The model under review builds one solid part; all positions refer to its coordinate system, in mm. A direction names the side the tool comes from. Coordinates: 2 decimals unless noted, no trailing zeros. Use one line per item in the form item = value. Start each with the question number.
(1) Insertion check: pin 1 Ø6 at (x, z) = (1, -8) entering from +Y; pin 2 Ø2 at (y, z) = (10, -5.5) entering from +X; pin 3 Ø1 at (x, y) = (-17, 7.5) entering from -Z (3 decimals); pin 4 Ø4 at (x, y) = (12.5, 8.5) entering from -Z. Each pin has a flat end and moves straight along its axis. Give the tip position at first contact, or say it passes through.
(2) For faces 5 (the cylindrical face through (-0.764, 0.724, 16.364)), 6 (the flat face through (-15.3, 10.795, 2.4)), 7 (the flat face through (0, 8, 16)), list the 3-axis set-ups (+Z, -Z, +X, -X, +Y, -Y) from which the entire face can be reached by the end or side of a thin tool; tool diameter is ignored.
(3) Take a section at A-A (x = -3.5). State how many separate pieces and enclosed holes the cut face has, then the cut area to 3 significant figures.
(4) Wall thickness on line 1 along X through (y, z) = (7.25, 6); line 2 along X through (y, z) = (7.5, 1.5); line 3 along Z through (x, y) = (-36, 6): over which ranges is each line inside the solid? List them lowest first.
(5) Mouldability with a two-part tool opening along Z and no side actions: class faces 1 (the flat face through (-39.597, 6.261, -10.359)), 2 (the cylindrical face through (-23.17, 0.72, 6.88)), 3 (the flat face through (-15.426, 6.261, -17.565)), 4 (the cylindrical face through (-15.374, 1.279, 3.601)) as +Z half, -Z half, draft (parallel to the pull), parting line (faces both ways), or undercut.
```python
from build123d import *

# Parameters (mm, degrees)
SKETCH1_W           = 16.825477707
SKETCH1_H           = 12.7
BOSS_EXTRUDE1_DEPTH = 12.7
FILLET1_R           = 7.62
SKETCH2_R           = 1.905
CUT_EXTRUDE1_DEPTH  = 12.7
SKETCH3_W           = 6.35
SKETCH3_H           = 12.7
BOSS_EXTRUDE2_DEPTH = 9.652
FILLET2_R           = 7.62
SKETCH4_R           = 1.905
CUT_EXTRUDE2_DEPTH  = 12.7
FILLET3_R           = 2.54
SKETCH5_W           = 1.27
SKETCH5_H           = 1.27
FILLET4_R           = 2.54


with BuildPart() as part:
    # Sketch1 → Boss-Extrude1 (new body)
    with BuildSketch(Plane(origin=(0, 0, 0), x_dir=(1, 0, 0), z_dir=(0, 1, 0))):
        Polygon((-42.597094971, 9.46433121), (0, 22.16433121), (0, -28.63566879), align=None)
        with Locations((8.412738854, -3.23566879)):
            Rectangle(SKETCH1_W, SKETCH1_H)
    extrude(amount=BOSS_EXTRUDE1_DEPTH)

    # Fillet1
    fillet1_edges = [part.edges().sort_by_distance(p)[0] for p in [
        (16.825477707, 0, 3.23566879),
    ]]
    fillet(fillet1_edges, radius=FILLET1_R)

    # Sketch2 → Cut-Extrude1 (cut)
    with BuildSketch(Plane.XY.offset(9.58566879)):
        with Locations((10.475477707, 6.35)):
            Circle(SKETCH2_R)
    extrude(amount=-CUT_EXTRUDE1_DEPTH, mode=Mode.SUBTRACT)

    # Sketch3 → Boss-Extrude2 (add)
    with BuildSketch(Plane(origin=(-6.06868791, 0, -20.35499805), x_dir=(-0.9583148474999098, 0, 0.2857142857142858), z_dir=(-0.2857142857142858, 0, -0.9583148474999098))):
        with Locations((28.59233394, 6.35)):
            Rectangle(SKETCH3_W, SKETCH3_H)
    extrude(amount=BOSS_EXTRUDE2_DEPTH)

    # Fillet2
    fillet2_edges = [part.edges().sort_by_distance(p)[0] for p in [
        (-36.226860335, 0, -21.43541469),
    ]]
    fillet(fillet2_edges, radius=FILLET2_R)

    # Sketch4 → Cut-Extrude2 (cut)
    with BuildSketch(Plane(origin=(-30.44310778, 0, 9.076381126), x_dir=(0.2857142857142858, 0, 0.9583148474999098), z_dir=(-0.9583148474999098, 0, 0.2857142857142858))):
        with Locations((-26.066407684, 6.604)):
            Circle(SKETCH4_R)
    extrude(amount=-CUT_EXTRUDE2_DEPTH, mode=Mode.SUBTRACT)

    # Fillet3
    fillet3_edges = [part.edges().sort_by_distance(p)[0] for p in [
        (0, 6.35, 28.63566879),
    ]]
    fillet(fillet3_edges, radius=FILLET3_R)

    # Sketch5 → Cut-Revolve1 (revolve, cut)
    with BuildSketch(Plane(origin=(-8.826402195, 0, -29.604652958), x_dir=(-0.9583148474999099, 0, 0.28571428571428553), z_dir=(-0.28571428571428553, 0, -0.9583148474999099))):
        with Locations((28.59233394, 11.43)):
            Rectangle(SKETCH5_W, SKETCH5_H)
        with Locations((28.59233394, 1.27)):
            Rectangle(SKETCH5_W, SKETCH5_H)
    revolve(axis=Axis((1.537963556, 18.050379457, -32.694709807), (0, -1, 0)), mode=Mode.SUBTRACT)

    # Fillet4
    fillet4_edges = [part.edges().sort_by_distance(p)[0] for p in [
        (0, 0, 16.270862458),
        (-23.415214152, 0, 7.692464569),
        (-1.503049342, 0, 25.274748287),
    ]]
    fillet(fillet4_edges, radius=FILLET4_R)


solid = part.part
```
Findings:
q1.pin_1 = 12.7
q1.pin_2 = 0
q1.pin_3 = -17.245
q1.pin_4 = -3.11
q2.face_5 = +Z, +X, -Y
q2.face_6 = none
q2.face_7 = +Z, +X, +Y, -Y
q3.separate_pieces = 1
q3.enclosed_holes = 2
q3.area = 585 mm²
q4.line_1 = -25.31 to 8.8, 12.15 to 16.82
q4.line_2 = -30.34 to 8.96, 11.99 to 16.82
q4.line_3 = -21.32 to -18.35, -14.58 to -3.56
q5.face_1 = undercut
q5.face_2 = +Z half
q5.face_3 = -Z half
q5.face_4 = undercut
